Geometry check sheet. Reference: the model listing, model coordinates, mm. A direction names the side the tool comes from. Coordinates: 2 decimals unless noted, no trailing zeros. Write each loop counter-clockwise with the first axis right and the second up, starting at its lowest first coordinate (ties: lowest second). Pieces come first, ordered by that corner, then holes.
from build123d import *


with BuildPart() as part:
    # SK_P01_Wheel125x30 → P01_Wheel125x30 (revolve)
    with BuildSketch(Plane(origin=(0, 62.5, 0), x_dir=(1, 0, 0), z_dir=(0, 1, 0)), mode=Mode.PRIVATE) as p01_wheel125x30_sk:
        Polygon((0, 15), (15, 15), (15, 10), (47, 10), (47, 15), (62.5, 15), (62.5, -15), (47, -15), (47, -10), (15, -10), (15, -15), (0, -15), align=None)
    revolve(p01_wheel125x30_sk.sketch.rotate(Axis((0, 62.5, -20), (0, 0, 1)), 180), axis=Axis((0, 62.5, -20), (0, 0, 1)))


solid = part.part
1. Sectioned sample at B-B, the plane x = 0. Record the boundary of the cut face in (y, z).
Computed values:
outline: (0, -15) - (15.5, -15) - (15.5, -10) - (47.5, -10) - (47.5, -15) - (77.5, -15) - (77.5, -10) - (109.5, -10) - (109.5, -15) - (125, -15) - (125, 15) - (109.5, 15) - (109.5, 10) - (77.5, 10) - (77.5, 15) - (47.5, 15) - (47.5, 10) - (15.5, 10) - (15.5, 15) - (0, 15) - close
2. Sectioned sample at A-A, the plane y = 62.5. Record the boundary of the cut face in (x, z), and give its area (3 significant figures).
Computed values:
outline: (-62.5, -15) - (-47, -15) - (-47, -10) - (-15, -10) - (-15, -15) - (15, -15) - (15, -10) - (47, -10) - (47, -15) - (62.5, -15) - (62.5, 15) - (47, 15) - (47, 10) - (15, 10) - (15, 15) - (-15, 15) - (-15, 10) - (-47, 10) - (-47, 15) - (-62.5, 15) - close
area: 3,110 mm2
3. Gauge pin test, flat ends, axial feed: pin 1 Ø4 at (y, z) = (105, -12) entering from +X; pin 2 Ø1.5 at (x, z) = (32.5, -5.5) entering from +Y; pin 3 Ø2 at (x, z) = (15.5, 10.5) entering from -Y. Record the tip position at first contact, or that the pin passes through.
Computed values:
pin 1: stops at x = 47.6
pin 2: stops at y = 116.33
pin 3: stops at y = 1.71
4. Thickness scan on line 1 along Y through (x, z) = (0, -13.55); line 2 along Z through (x, y) = (15, 18); line 3 along Y through (x, z) = (35.5, 9). Record the ranges inside material, lowest first.
Computed values:
line 1: y = 0 to 15.5, 47.5 to 77.5, 109.5 to 125
line 2: z = -10 to 10
line 3: y = 11.06 to 113.94
5. Sectioned sample at D-D, the plane y = 42.5. Record the boundary of the cut face in (x, z), and give its area (3 significant figures).
Computed values:
outline: (-59.21, -15) - (-42.53, -15) - (-42.53, -10) - (42.53, -10) - (42.53, -15) - (59.21, -15) - (59.21, 15) - (42.53, 15) - (42.53, 10) - (-42.53, 10) - (-42.53, 15) - (-59.21, 15) - close
area: 2,700 mm2
6. Draft check along Y on faces 1 (the cylindrical face through (8.136, 0.532, 0.21)), 2 (the flat face through (0, 62, 15)), 3 (the cylindrical face through (3.252, 77.143, -12.465)). Enter one of: released by +Y, released by -Y, zero draft, split by the parting line, or undercut.
Computed values:
face 1: split by the parting line
face 2: zero draft
face 3: undercut
7. Sectioned sample at C-C, the plane z = 3. Record the boundary of the cut face in (x, y), and give its area (3 significant figures).
Computed values:
outline: circle Ø125 at (0, 62.5)
area: 12,300 mm2
8. Access from +Z, -Z, +X, -X, +Y, -Y to the whole of each face (thin tool, end or side, straight path). Record for faces 4 (the cylindrical face through (-21.688, 104.197, 12.465)), 5 (the flat face through (-9, 16, 15)), 6 (the flat face through (-11, 51, -10)).
Computed values:
face 4: +Z
face 5: +Z, +X, -X, +Y, -Y
face 6: -Z
